The listing builds one solid part. Answer for the finished solid, in the listing's coordinates (mm). A direction names the side the tool comes from. Give positions to 0.01 mm unless a question says otherwise; leave off trailing zeros. Write each loop counter-clockwise with the first axis right and the second up, starting at its lowest first coordinate (ties: lowest second). Pieces come first, ordered by that corner, then holes. Notation, with made-up numbers: (14, -24) -> (25, -24) arc R23 cw to (25, -2) -> close; hole circle Ø11 at (-34, -19.75). An arc over 180 degrees is marked (long way). One line per question, with ' | ' between items.
from build123d import *

# Parameters (mm, degrees)
EXTRUDE_1_DEPTH          = 27.2
SKETCH_2_R               = 15
EXTRUDE_2_DEPTH          = 0.1
SKETCH_3_R               = 1.7
CUT_EXTRUDE_2_DEPTH      = 41
SKETCH_4_R               = 5
CUT_EXTRUDE_3_DEPTH      = 41
SKETCH_6_R               = 5
SKETCH_6_R_2             = 1.7
CUT_EXTRUDE_4_DEPTH      = 60
SKETCH_8_R               = 3.7
CUT_EXTRUDE_5_DEPTH      = 11.2
CUT_EXTRUDE_6_DEPTH      = 40
CUT_EXTRUDE_7_DEPTH      = 14.5
CUT_EXTRUDE_7_DEPTH_BACK = 12.7
SKETCH_24_R              = 3.7
FILLET_1_R               = 10
SKETCH_25_W              = 104
SKETCH_25_H              = 148.506502633
CUT_EXTRUDE_8_DEPTH      = 3
SKETCH_26_W              = 84
SKETCH_26_H              = 40
CUT_EXTRUDE_9_DEPTH      = 5
SKETCH_27_R              = 1.7
CUT_EXTRUDE_10_DEPTH     = 55
CUT_EXTRUDE_11_DEPTH     = 7.2


with BuildPart() as part:
    # 草图1 → 凸台-拉伸1 (new body)
    with BuildSketch(Plane(origin=(0, 0, 0), x_dir=(1, 0, 0), z_dir=(0, 1, 0))):
        with BuildLine():
            Line((0, 28.5), (220, 28.5))
            Line((220, 28.5), (220, -28.5))
            Line((220, -28.5), (0, -28.5))
            ThreePointArc((0, -28.5), (-28.5, 0), (0, 28.5))
        make_face()
    extrude(amount=EXTRUDE_1_DEPTH)

    # 草图2 → 凸台-拉伸2 (add)
    with BuildSketch(Plane(origin=(0, 27.2, 0), x_dir=(1, 0, 0), z_dir=(0, 1, 0))):
        with Locations(Location((0, 0, 0), (0, 0, 270))):
            Circle(SKETCH_2_R)
    extrude(amount=EXTRUDE_2_DEPTH)

    # 草图3 → 切除-拉伸2 (cut)
    with BuildSketch(Plane(origin=(0, 27.3, 0), x_dir=(1, 0, 0), z_dir=(0, 1, 0))):
        with Locations(Location((0, 13.5, 0), (0, 0, 270))):
            Circle(SKETCH_3_R)
        with Locations(Location((11.691342951, 6.75, 0), (0, 0, 270))):
            Circle(SKETCH_3_R)
        with Locations(Location((11.691342951, -6.75, 0), (0, 0, 270))):
            Circle(SKETCH_3_R)
        with Locations(Location((0, -13.5, 0), (0, 0, 270))):
            Circle(SKETCH_3_R)
        with Locations(Location((-11.691342951, -6.75, 0), (0, 0, 270))):
            Circle(SKETCH_3_R)
        with Locations(Location((-11.691342951, 6.75, 0), (0, 0, 270))):
            Circle(SKETCH_3_R)
    extrude(amount=-CUT_EXTRUDE_2_DEPTH, mode=Mode.SUBTRACT)

    # 草图4 → 切除-拉伸3 (cut)
    with BuildSketch(Plane(origin=(0, 27.3, 0), x_dir=(1, 0, 0), z_dir=(0, 1, 0))):
        with Locations(Location((0, 0, 0), (0, 0, 270))):
            Circle(SKETCH_4_R)
    extrude(amount=-CUT_EXTRUDE_3_DEPTH, mode=Mode.SUBTRACT)

    # 草图6 → 切除-拉伸4 (cut)
    with BuildSketch(Plane(origin=(0, 27.2, 0), x_dir=(1, 0, 0), z_dir=(0, 1, 0))):
        with Locations(Location((184, 0, 0), (0, 0, 270))):
            Circle(SKETCH_6_R)
        with Locations(Location((184, 19, 0), (0, 0, 270))):
            Circle(SKETCH_6_R_2)
        with Locations(Location((165, 0, 0), (0, 0, 270))):
            Circle(SKETCH_6_R_2)
        with Locations(Location((184, -19, 0), (0, 0, 270))):
            Circle(SKETCH_6_R_2)
        with Locations(Location((203, 0, 0), (0, 0, 270))):
            Circle(SKETCH_6_R_2)
    extrude(amount=-CUT_EXTRUDE_4_DEPTH, mode=Mode.SUBTRACT)

    # 草图8 → 切除-拉伸5 (cut)
    with BuildSketch(Plane(origin=(0, 27.2, 0), x_dir=(1, 0, 0), z_dir=(0, 1, 0))):
        with Locations(Location((184, 19, 0), (0, 0, 270))):
            Circle(SKETCH_8_R)
        with Locations(Location((203, 0, 0), (0, 0, 270))):
            Circle(SKETCH_8_R)
        with Locations(Location((184, -19, 0), (0, 0, 270))):
            Circle(SKETCH_8_R)
        with Locations(Location((165, 0, 0), (0, 0, 270))):
            Circle(SKETCH_8_R)
    extrude(amount=-CUT_EXTRUDE_5_DEPTH, mode=Mode.SUBTRACT)

    # 草图20 → 切除-拉伸6 (cut)
    with BuildSketch(Plane(origin=(0, 27.2, 0), x_dir=(1, 0, 0), z_dir=(0, 1, 0))):
        with BuildLine():
            Line((184, 28.5), (231.029995119, 28.5))
            Line((231.029995119, 28.5), (231.029995119, -33.501225727))
            Line((231.029995119, -33.501225727), (184, -33.501225727))
            Line((184, -33.501225727), (184, -28.5))
            ThreePointArc((184, -28.5), (212.5, 0), (184, 28.5))
        make_face()
    extrude(amount=-CUT_EXTRUDE_6_DEPTH, mode=Mode.SUBTRACT)

    # 草图24 → 切除-拉伸7 (cut, two sides: drawn at the far end of the back side and taken through both)
    with BuildSketch(Plane(origin=(0, 27.2, 0), x_dir=(1, 0, 0), z_dir=(0, 1, 0)).offset(-CUT_EXTRUDE_7_DEPTH_BACK)):
        with Locations(Location((0, -13.5, 0), (0, 0, 343.088700116))):
            Circle(SKETCH_24_R)
        with Locations(Location((-11.691342951, -6.75, 0), (0, 0, 136.911299884))):
            Circle(SKETCH_24_R)
        with Locations(Location((-11.691342951, 6.75, 0), (0, 0, 76.911299884))):
            Circle(SKETCH_24_R)
        with Locations(Location((0, 13.5, 0), (0, 0, 16.911299884))):
            Circle(SKETCH_24_R)
        with Locations(Location((11.691342951, 6.75, 0), (0, 0, 103.088700116))):
            Circle(SKETCH_24_R)
        with Locations(Location((11.691342951, -6.75, 0), (0, 0, 43.088700116))):
            Circle(SKETCH_24_R)
    extrude(amount=CUT_EXTRUDE_7_DEPTH + CUT_EXTRUDE_7_DEPTH_BACK, mode=Mode.SUBTRACT)

    # 圆角1
    # the kernel refuses this fillet: 10 mm, written as the material it takes off along each edge
    with BuildSketch(Plane(origin=(0, 27.2, -28.5), x_dir=(0, -1, 0), z_dir=(1, 0, 0))) as fillet_1_piece_1:
        with BuildLine():
            CenterArc((FILLET_1_R, -FILLET_1_R), FILLET_1_R, 90, 90)
            Line((0, -FILLET_1_R), (0, 0))
            Line((0, 0), (FILLET_1_R, 0))
        make_face()
    extrude(amount=184, mode=Mode.SUBTRACT)
    with BuildSketch(Plane(origin=(184, 27.2, 0), x_dir=(0, 0, 1), z_dir=(-1, 0, 0))) as fillet_1_piece_2:
        with BuildLine():
            CenterArc((28.5 - FILLET_1_R, -FILLET_1_R), FILLET_1_R, 0, 90)
            Line((28.5 - FILLET_1_R, 0), (28.5, 0))
            Line((28.5, 0), (28.5, -FILLET_1_R))
        make_face()
    revolve(axis=Axis((184, 27.2, 0), (0, 1, 0)), revolution_arc=180, mode=Mode.SUBTRACT)
    with BuildSketch(Plane(origin=(0, 27.2, 0), x_dir=(0, 0, 1), z_dir=(1, 0, 0))) as fillet_1_piece_3:
        with BuildLine():
            CenterArc((28.5 - FILLET_1_R, FILLET_1_R), FILLET_1_R, 270, 90)
            Line((28.5, FILLET_1_R), (28.5, 0))
            Line((28.5, 0), (28.5 - FILLET_1_R, 0))
        make_face()
    revolve(axis=Axis((0, 27.2, 0), (0, -1, 0)), revolution_arc=180, mode=Mode.SUBTRACT)
    with BuildSketch(Plane(origin=(184, 27.2, 28.5), x_dir=(0, 0, -1), z_dir=(-1, 0, 0))) as fillet_1_piece_4:
        with BuildLine():
            CenterArc((FILLET_1_R, FILLET_1_R), FILLET_1_R, 180, 90)
            Line((0, FILLET_1_R), (0, 0))
            Line((0, 0), (FILLET_1_R, 0))
        make_face()
    extrude(amount=184, mode=Mode.SUBTRACT)

    # 草图25 → 切除-拉伸8 (cut)
    with BuildSketch(Plane.XZ):
        with Locations((92, -1.302688619)):
            Rectangle(SKETCH_25_W, SKETCH_25_H)
    extrude(amount=-CUT_EXTRUDE_8_DEPTH, mode=Mode.SUBTRACT)

    # 草图26 → 切除-拉伸9 (cut)
    with BuildSketch(Plane.XZ.offset(-3)):
        with Locations((92, 0)):
            Rectangle(SKETCH_26_W, SKETCH_26_H)
    extrude(amount=-CUT_EXTRUDE_9_DEPTH, mode=Mode.SUBTRACT)

    # 草图27 → 切除-拉伸10 (cut)
    with BuildSketch(Plane.XZ.offset(-3)):
        with Locations(Location((45, 0, 0), (0, 0, 270))):
            Circle(SKETCH_27_R)
        with Locations(Location((139, 0, 0), (0, 0, 270))):
            Circle(SKETCH_27_R)
    extrude(amount=-CUT_EXTRUDE_10_DEPTH, mode=Mode.SUBTRACT)

    # 草图28 → 切除-拉伸11 (cut)
    with BuildSketch(Plane(origin=(0, 27.2, 0), x_dir=(1, 0, 0), z_dir=(0, 1, 0))):
        Polygon((41.824573519, 0), (43.41228676, -2.75), (46.58771324, -2.75), (48.175426481, 0), (46.58771324, 2.75), (43.41228676, 2.75), align=None)
        Polygon((135.824573519, 0), (137.41228676, -2.75), (140.58771324, -2.75), (142.175426481, 0), (140.58771324, 2.75), (137.41228676, 2.75), align=None)
    extrude(amount=-CUT_EXTRUDE_11_DEPTH, mode=Mode.SUBTRACT)


solid = part.part
Item 1: Find section B-B (y = 12.5). Count the separate pieces of the cut face and the enclosed holes in it, then the cut area to 3 significant figures.
Answers below:
separate pieces: 1 | enclosed holes: 14 | area: 12,800 mm²
Item 2: Determine the mould class of faces 1 (the face through (91, 8, -28.5)), 2 (the face through (212.493, 8.72, 0.627)), 3 (the face through (-4.88, 13.84, -1.08)) for opening direction X: pulls with the +X half, pulls with the -X half, needs draft (parallel to the pull), parting line crosses it, or undercut.
Answers below:
face 1: needs draft | face 2: pulls with the +X half | face 3: undercut
Item 3: A tool of negligible diameter and unlimited length cuts with its end or side. For faces 4 (the face through (91, 5, -20)), 5 (the face through (9.81, 20.81, -9.936)), from which of +Z, -Z, +X, -X, +Y, -Y can it reach the whole face along a straight path? Write none if from no direction.
Answers below:
face 4: -Y | face 5: +Y
Item 4: Flat-ended cylindrical pins translate along their axes: pin 1 (10 mm diameter, centred on y = 17, z = 5, fed in from +X); pin 2 (1 mm diameter, centred on y = 23, z = 10, fed in from +X); pin 3 (5 mm diameter, centred on x = 54.5, z = -20.5, fed in from -Y); pin 4 (2 mm diameter, centred on x = -11.69, z = -6.75, fed in from +Y). Find the tip coordinate at first contact, or state that the pin passes through.
Answers below:
pin 1: x = 212.5 | pin 2: x = 209.11 | pin 3: y = 3 | pin 4: through
Item 5: Find section C-C (x = 156). Write down the section's boundary in (y, z).
Answers below:
outline: (0, -28.5) -> (17.2, -28.5) arc R10 ccw to (27.2, -18.5) -> (27.2, 18.5) arc R10 ccw to (17.2, 28.5) -> (0, 28.5) -> close
Item 6: Consider line 1 (Z direction, x = 115.5, y = 4); line 2 (X direction, y = 3.25, z = 18); line 3 (X direction, y = 22.5, z = 6.75). Determine where each line is inside the solid, lowest interval first. Write a range as [from, to].
Answers below:
line 1: [-28.5, -20], [20, 28.5] | line 2: [-22.1, 50], [134, 182.63], [185.37, 206.1] | line 3: [-26.12, -15.39], [-7.99, 7.99], [15.39, 210.12]
Item 7: Find section A-A (x = 89). Write down the section's boundary in (y, z), then the cut area to 3 significant figures.
Answers below:
outline: (3, -28.5) -> (17.2, -28.5) arc R10 ccw to (27.2, -18.5) -> (27.2, 18.5) arc R10 ccw to (17.2, 28.5) -> (3, 28.5) -> (3, 20) -> (8, 20) -> (8, -20) -> (3, -20) -> close | area: 1,140 mm²
